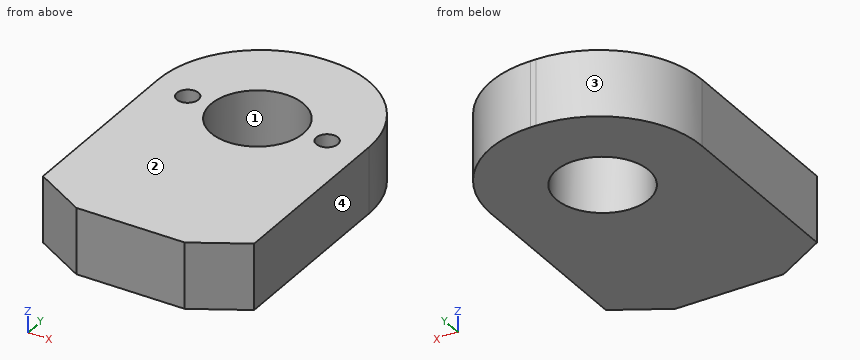
```python
from build123d import *

# Parameters (mm, degrees)
SKETCH2_R           = 6.3
BOSS_EXTRUDE1_DEPTH = 9
SKETCH3_R           = 1.475
CUT_EXTRUDE1_DEPTH  = 4


with BuildPart() as part:
    # Sketch2 → Boss-Extrude1 (new body)
    with BuildSketch(Plane.XY):
        with BuildLine():
            Line((0, 4), (7, 0))
            Line((7, 0), (21.77, 0))
            Line((21.77, 0), (28.77, 4))
            Line((28.77, 4), (28.77, 29.38))
            ThreePointArc((28.77, 29.38), (24.669494937, 39.279494937), (14.77, 43.38))
            Line((14.77, 43.38), (14, 43.38))
            ThreePointArc((14, 43.38), (4.100505063, 39.279494937), (0, 29.38))
            Line((0, 29.38), (0, 4))
        make_face()
        with Locations((14.385, 28.04)):
            Circle(SKETCH2_R, mode=Mode.SUBTRACT)
    extrude(amount=BOSS_EXTRUDE1_DEPTH)

    # Sketch3 → Cut-Extrude1 (cut)
    with BuildSketch(Plane.XY.offset(9)):
        with Locations((4.885, 28.04)):
            Circle(SKETCH3_R)
        with Locations((23.885, 28.04)):
            Circle(SKETCH3_R)
    extrude(amount=-CUT_EXTRUDE1_DEPTH, mode=Mode.SUBTRACT)


solid = part.part
```
Input: part model. Units: mm. Frame: model coordinates. Face numbers are marked on the shaded views. Round coordinates to 2 decimals unless told otherwise and drop trailing zeros. Loops run counter-clockwise (first coordinate to the right, second up) from the corner with the lowest first, then second, coordinate; pieces in that order, holes last.
1) Pin query (flat end, axial travel): pin 1 (4 mm diameter, centred on y = 14, z = 4, fed in from -X); pin 2 (1.8 mm diameter, centred on x = 4.885, y = 28.04, fed in from +Z); pin 3 (1.5 mm diameter, centred on x = 19, y = 25.5, fed in from -Z); pin 4 (2 mm diameter, centred on x = 20.5, z = 2.5, fed in from +Y). Return the tip coordinate at first contact, or that it passes through.
Ans:
pin 1: stops at x = 0
pin 2: stops at z = 5
pin 3: passes through
pin 4: stops at y = 42.56
2) Section query B-B on y = 28.04. Return the cut outline in (x, z) (3 decimals), plus the area to 3 significant figures.
Ans:
outline: (0, 0) - (8.085, 0) - (8.085, 9) - (6.36, 9) - (6.36, 5) - (3.41, 5) - (3.41, 9) - (0, 9) - close; (20.685, 0) - (28.77, 0) - (28.77, 9) - (25.36, 9) - (25.36, 5) - (22.41, 5) - (22.41, 9) - (20.685, 9) - close
area: 122 mm2
3) Section query C-C on x = 13. Return the cut outline in (y, z).
Ans:
outline: (0, 0) - (21.89, 0) - (21.89, 9) - (0, 9) - close; (34.19, 0) - (43.34, 0) - (43.34, 9) - (34.19, 9) - close
4) Material intervals for line 1 (Y direction, x = 14.75, z = 7.5); line 2 (X direction, y = 41.5, z = 4.5); line 3 (Y direction, x = 9.5, z = 2.75), sorted ascending.
Ans:
line 1: y = 0 to 21.75, 34.33 to 43.38
line 2: x = 6.99 to 21.78
line 3: y = 0 to 24.06, 32.02 to 42.64
5) Section query D-D on z = 1.5. Return the cut outline in (x, y) (3 decimals).
Ans:
outline: (0, 4) - (7, 0) - (21.77, 0) - (28.77, 4) - (28.77, 29.38) arc R14 ccw to (14.77, 43.38) - (14, 43.38) arc R14 ccw to (0, 29.38) - close; hole circle Ø12.6 at (14.385, 28.04)
6) Section query A-A on z = 5.5. Return the cut outline in (x, y) (3 decimals).
Ans:
outline: (0, 4) - (7, 0) - (21.77, 0) - (28.77, 4) - (28.77, 29.38) arc R14 ccw to (14.77, 43.38) - (14, 43.38) arc R14 ccw to (0, 29.38) - close; hole circle Ø2.95 at (4.885, 28.04); hole circle Ø12.6 at (14.385, 28.04); hole circle Ø2.95 at (23.885, 28.04)
7) Pull-direction query (X, two-part tool) for the marked faces 1, 2, 3 and 4; classes: released by +X, released by -X, zero draft, split by the parting line, or undercut.
Ans:
face 1: undercut
face 2: zero draft
face 3: released by -X
face 4: released by +X
